For this review, take the finished solid that the model builds, in its own axes (mm). A direction names the side the tool comes from. Round coordinates to 2 decimals unless told otherwise and drop trailing zeros. Order: outer loops, then holes, each group sorted by start corner. A loop starts at its lowest first (then second) coordinate and runs counter-clockwise, first axis right, second up. Notation, with made-up numbers: (8, -9.75) -> (17, -9.75) arc R28 ccw to (17, 29.25) -> close; hole circle Ø2 at (-29, 52). An arc over 180 degrees is marked (long way). Put each result on its own line as item: value. Start each with the question number.
```python
from build123d import *

# Parameters (mm, degrees)
F0_W     = 116
F0_H     = 94
F1_DEPTH = 8
F3_D     = 7.9
F3_DEPTH = 5
F3_TIP   = 2.3733994452
F5_D     = 2.5
F6_R     = 5


with BuildPart() as f1:
    # F0 (on Top) → F1 (new body)
    with BuildSketch(Plane.XY):
        Rectangle(F0_W, F0_H)
    extrude(amount=F1_DEPTH)

    # F3
    with Locations(Plane.XY.offset(8)):
        with Locations((-44, 33), (-22, 20), (-44, 7), (-44, -19), (-22, -6), (0, -19), (0, 7), (0, 33), (22, 20), (22, -6), (44, 7), (44, 33), (44, -19)):
            Hole(F3_D / 2, depth=F3_DEPTH)
            with Locations((0, 0, -(F3_DEPTH + F3_TIP / 2))):  # 118° drill point
                Cone(0, F3_D / 2, F3_TIP, mode=Mode.SUBTRACT)

    # F5 (through all)
    with Locations(Plane.XY.offset(8)):
        with Locations((-50, -41), (50, -41)):
            Hole(F5_D / 2)

    # F6
    f6_edges = [f1.edges().sort_by_distance(p)[0] for p in [
        (-58, -47, 4),
        (58, -47, 4),
        (-58, 47, 4),
        (58, 47, 4),
    ]]
    fillet(f6_edges, radius=F6_R)


solid = f1.part
```
Item 1: Mouldability with a two-part tool opening along Y and no side actions: class faces 3 (the face through (-1, -47, 4)), 4 (the face through (-1, 1, 0)), 5 (the face through (40.232, 8.186, 5.465)) as +Y half, -Y half, draft (parallel to the pull), parting line (faces both ways), or undercut.
Item 2: Consider section B-B, the plane z = 5.25. Count the separate pieces of the cut face and the enclosed holes in it, plus the area to 3 significant figures.
Item 3: Tool access review of faces 1 (the face through (-1, 47, 4)), 2 (the face through (40.35, -20.51, 5.46)): name each direction out of +Z, -Z, +X, -X, +Y, -Y from which nothing blocks a thin tool from reaching the whole face with its end or side.
Item 4: Consider section A-A, the plane x = 50. Write out the cut boundary in (y, z).
Item 5: For L1, parallel to X at y = -6, z = 4.25; L2, parallel to Y at x = -44, z = 5.7; L3, parallel to X at y = -19, z = 5.85, list the stretches that pass through material, from the lowest coordinate up.
Item 6: Insertion check: pin 1 Ø10 at (x, y) = (-42, 18) entering from -Z; pin 2 Ø4.5 at (x, y) = (0, -19) entering from +Z; pin 3 Ø1.5 at (x, y) = (50, -41) entering from +Z; pin 4 Ø6.5 at (x, y) = (-22, -6) entering from +Z. Each pin has a flat end and moves straight along its axis. Give the tip position at first contact, or say it passes through.
Evaluation:
1. face 3: -Y half
1. face 4: draft
1. face 5: undercut
2. separate pieces: 1
2. enclosed holes: 15
2. area: 10,200 mm^2
3. face 1: +Z, -Z, +X, -X, +Y
3. face 2: +Z
4. outline: (-47, 0) -> (-42.25, 0) -> (-42.25, 8) -> (-47, 8) -> close; (-39.75, 0) -> (47, 0) -> (47, 8) -> (-39.75, 8) -> close
5. L1: x = -58 to -25.95, -18.05 to 18.05, 25.95 to 58
5. L2: y = -47 to -22.95, -15.05 to 3.05, 10.95 to 29.05, 36.95 to 47
5. L3: x = -58 to -47.95, -40.05 to -3.95, 3.95 to 40.05, 47.95 to 58
6. pin 1: stops at z = 0
6. pin 2: stops at z = 1.98
6. pin 3: passes through
6. pin 4: stops at z = 2.58
